```python
from build123d import *

# Parameters (mm, degrees)
SKETCH1_W           = 25.4
SKETCH1_H           = 25.4
BOSS_EXTRUDE1_DEPTH = 8.89
SKETCH2_R           = 1.9939
SKETCH2_R_2         = 2.032
BOSS_EXTRUDE2_DEPTH = 11.303
SKETCH3_R           = 1.6383
CUT_EXTRUDE1_DEPTH  = 21.193


with BuildPart() as part:
    # Sketch1 → Boss-Extrude1 (new body)
    with BuildSketch(Plane(origin=(0, 0, 0), x_dir=(1, 0, 0), z_dir=(0, 1, 0))):
        with Locations((-4.163944862, -1.223942607)):
            Rectangle(SKETCH1_W, SKETCH1_H)
    extrude(amount=BOSS_EXTRUDE1_DEPTH)

    # Sketch2 → Boss-Extrude2 (add)
    with BuildSketch(Plane.XZ):
        with Locations((-14.577944862, 11.637942607)):
            Circle(SKETCH2_R)
        with Locations((6.250055138, 11.637942607)):
            Circle(SKETCH2_R_2)
        with Locations((6.250055138, -9.190057393)):
            Circle(SKETCH2_R_2)
        with Locations((-14.577944862, -9.190057393)):
            Circle(SKETCH2_R_2)
    extrude(amount=BOSS_EXTRUDE2_DEPTH)

    # Sketch3 → Cut-Extrude1 (cut, through all)
    with BuildSketch(Plane.XZ.offset(11.303)):
        with Locations((-14.577944862, 11.637942607)):
            Circle(SKETCH3_R)
        with Locations((-14.577944862, -9.190057393)):
            Circle(SKETCH3_R)
        with Locations((6.250055138, -9.190057393)):
            Circle(SKETCH3_R)
        with Locations((6.250055138, 11.637942607)):
            Circle(SKETCH3_R)
    extrude(amount=-CUT_EXTRUDE1_DEPTH, mode=Mode.SUBTRACT)


solid = part.part
```
Model file for the job. Use its own axes, mm. A direction names the side the tool comes from. Give positions to 0.01 mm unless a question says otherwise; leave off trailing zeros. Order: outer loops, then holes, each group sorted by start corner. A loop starts at its lowest first (then second) coordinate and runs counter-clockwise, first axis right, second up.
1) Mould opens along X. For faces 3 (the cylindrical face through (-12.676, -5.572, 12.237)), 4 (the flat face through (-16, -11.303, -8)), 5 (the flat face through (-16.864, 4, 1)) say: +X half, -X half, draft (parallel to the pull), parting line (faces both ways), or undercut.
2) Saw through at B-B, the plane y = -0.5. Write the cut outline in (x, z), then the cut area to 3 significant figures.
3) Saw through at A-A, the plane x = -14.25. Write the cut outline in (y, z), then the cut area to 3 significant figures.
4) Saw through at D-D, the plane x = 5.25. Write the cut outline in (y, z).
5) Saw through at C-C, the plane y = 7. Write the cut outline in (x, z), then the cut area to 3 significant figures.
6) Wall check: probe 1 along Z at (x, y) = (-15, 3); probe 2 along Y at (x, z) = (-4.5, 5); probe 3 along Z at (x, y) = (5, -7.25). Give the ranges that are in metal, low to high.
7) 3-axis set-ups, long thin cutter, end or side, ignore diameter. For faces 1 (the cylindrical face through (-12.7, -5.57, -9.97)), 2 (the cylindrical face through (7.13, -1.35, -7.81)): which of +Z, -Z, +X, -X, +Y, -Y reach the whole face in a straight line?
8) Pin check, flat tip, straight feed: pin 1 (5 mm diameter, centred on x = 1, z = 2.5, fed in from -Y). Stop position of the tip, or through.
Computed:
1. face 3: undercut
1. face 4: draft
1. face 5: -X half
2. outline: circle Ø4.06 at (-14.58, -9.19); circle Ø3.99 at (-14.58, 11.64); circle Ø4.06 at (6.25, -9.19); circle Ø4.06 at (6.25, 11.64); hole circle Ø3.28 at (-14.58, -9.19); hole circle Ø3.28 at (-14.58, 11.64); hole circle Ø3.28 at (6.25, -9.19); hole circle Ø3.28 at (6.25, 11.64)
2. area: 17.7 mm2
3. outline: (-11.3, -11.2) - (0, -11.2) - (0, -11.48) - (8.89, -11.48) - (8.89, -10.8) - (-11.3, -10.8) - close; (-11.3, -7.58) - (8.89, -7.58) - (8.89, 10.03) - (-11.3, 10.03) - (-11.3, 9.67) - (0, 9.67) - (0, -7.18) - (-11.3, -7.18) - close; (-11.3, 13.24) - (8.89, 13.24) - (8.89, 13.92) - (0, 13.92) - (0, 13.6) - (-11.3, 13.6) - close
3. area: 186 mm2
4. outline: (-11.3, -10.96) - (0, -10.96) - (0, -11.48) - (8.89, -11.48) - (8.89, -10.49) - (-11.3, -10.49) - close; (-11.3, -7.89) - (8.89, -7.89) - (8.89, 10.34) - (-11.3, 10.34) - (-11.3, 9.87) - (0, 9.87) - (0, -7.42) - (-11.3, -7.42) - close; (-11.3, 12.94) - (8.89, 12.94) - (8.89, 13.92) - (0, 13.92) - (0, 13.41) - (-11.3, 13.41) - close
5. outline: (-16.86, -11.48) - (8.54, -11.48) - (8.54, 13.92) - (-16.86, 13.92) - close; hole circle Ø3.28 at (-14.58, -9.19); hole circle Ø3.28 at (-14.58, 11.64); hole circle Ø3.28 at (6.25, -9.19); hole circle Ø3.28 at (6.25, 11.64)
5. area: 611 mm2
6. probe 1: z = -11.48 to -10.77, -7.61 to 10.05, 13.22 to 13.92
6. probe 2: y = 0 to 8.89
6. probe 3: z = -10.79 to -10.25, -8.13 to -7.59, 10.04 to 10.58, 12.7 to 13.24
7. face 1: -Y
7. face 2: +Y, -Y
8. pin 1: stops at y = 0
